```python
from build123d import *

# Parameters (mm, degrees)
SKETCH1_R           = 12.7
SKETCH1_R_2         = 1.35255
BOSS_EXTRUDE1_DEPTH = 4.445
SKETCH2_R           = 6.35
CUT_EXTRUDE1_DEPTH  = 0.762
CUT_EXTRUDE4_DEPTH  = 1.778
SKETCH6_R           = 1.8288
CUT_EXTRUDE5_DEPTH  = 2.905


with BuildPart() as part:
    # Sketch1 → Boss-Extrude1 (new body)
    with BuildSketch(Plane(origin=(0, 0, 0), x_dir=(0, 0, -1), z_dir=(1, 0, 0))):
        Circle(SKETCH1_R)
        with Locations((0, 9.779)):
            Circle(SKETCH1_R_2, mode=Mode.SUBTRACT)
        with Locations((6.914797213, 6.914797213)):
            Circle(SKETCH1_R_2, mode=Mode.SUBTRACT)
        with Locations((9.779, 0)):
            Circle(SKETCH1_R_2, mode=Mode.SUBTRACT)
        with Locations((6.914797213, -6.914797213)):
            Circle(SKETCH1_R_2, mode=Mode.SUBTRACT)
        with Locations((0, -9.779)):
            Circle(SKETCH1_R_2, mode=Mode.SUBTRACT)
        with Locations((-6.914797213, -6.914797213)):
            Circle(SKETCH1_R_2, mode=Mode.SUBTRACT)
        with Locations((-9.779, 0)):
            Circle(SKETCH1_R_2, mode=Mode.SUBTRACT)
        with Locations((-6.914797213, 6.914797213)):
            Circle(SKETCH1_R_2, mode=Mode.SUBTRACT)
    extrude(amount=BOSS_EXTRUDE1_DEPTH)

    # Sketch2 → Cut-Extrude1 (cut)
    with BuildSketch(Plane(origin=(4.445, 0, 0), x_dir=(0, 0, -1), z_dir=(1, 0, 0))):
        Circle(SKETCH2_R)
    extrude(amount=-CUT_EXTRUDE1_DEPTH, mode=Mode.SUBTRACT)

    # Sketch5 → Cut-Extrude4 (cut)
    with BuildSketch(Plane(origin=(3.683, 0, 0), x_dir=(0, 0, -1), z_dir=(1, 0, 0))):
        Polygon((-2.305627782, 3.948070989), (-4.571943663, -0.022696736), (-2.266315881, -3.970767725), (2.305627782, -3.948070989), (4.571943663, 0.022696736), (2.266315881, 3.970767725), align=None)
    extrude(amount=-CUT_EXTRUDE4_DEPTH, mode=Mode.SUBTRACT)

    # Sketch6 → Cut-Extrude5 (cut, through all)
    with BuildSketch(Plane(origin=(1.905, 0, 0), x_dir=(0, 0, -1), z_dir=(1, 0, 0))):
        Circle(SKETCH6_R)
    extrude(amount=-CUT_EXTRUDE5_DEPTH, mode=Mode.SUBTRACT)


solid = part.part
```
Model file for the job. Use its own axes, mm. A direction names the side the tool comes from. Round coordinates to 2 decimals unless told otherwise and drop trailing zeros. Loops run counter-clockwise (first coordinate to the right, second up) from the corner with the lowest first, then second, coordinate; pieces in that order, holes last. Notation, with made-up numbers: M 48,77.25 L 52,77.25 A25 cw 52,112.25 Z; hole C 48.5,-16.75 d3. An arc over 180 degrees is marked long. Put each result on its own line as item: value. Start each with the question number.
Item 1: Drill centre lines: line 1 along Z through (x, y) = (1.25, 6.75); line 2 along Z through (x, y) = (1.55, 7); line 3 along Y through (x, z) = (0.95, -0.5). Where is each one in solid material? Low to high.
Item 2: 3-axis set-ups, long thin cutter, end or side, ignore diameter. For faces 5 (the face through (2.806, 1.99, 3.423)), 6 (the face through (0, 0, -3)): which of +Z, -Z, +X, -X, +Y, -Y reach the whole face in a straight line?
Item 3: Cut at D-D (y = 4.75). List the corners of the cut face in (x, z) (3 decimals).
Item 4: Drop flat-ended pins along their axis: P1, Ø10, axis at y = -0.5, z = 0, coming from the +X side; P2, Ø1.5, axis at x = 3, y = 4.5, coming from the -Z side; P3, Ø2, axis at x = 2, y = 9.5, coming from the +Z side. Give the stop position or say it passes through.
Item 5: Mould opens along Y. For faces 1 (the face through (4.445, 6, -3)), 2 (the face through (2.19, -12.4, 2.75)), 3 (the face through (2.19, 0.41, -11.07)), 4 (the face through (2.806, -1.969, 3.435)) say: released by +Y, released by -Y, zero draft, split by the parting line, or undercut.
Item 6: Cut at B-B (z = 0). List the corners of the cut face in (x, y) (3 decimals).
Item 7: Cut at C-C (x = 3). Give the number of separate pieces and of enclosed holes in the cut face, then the cut area to 3 significant figures.
Item 8: Cut at A-A (y = -8.75). List the corners of the cut face in (x, z) (3 decimals).
Answer block:
1. line 1: -10.76 to -8.26, -5.57 to 5.57, 8.26 to 10.76
1. line 2: -10.6 to -8.26, -5.56 to 5.56, 8.26 to 10.6
1. line 3: -12.69 to -11.04, -8.52 to -1.76, 1.76 to 8.52, 11.04 to 12.69
2. face 5: +X
2. face 6: +Z, -Z, -X, +Y, -Y
3. outline: M 0,-11.778 L 4.445,-11.778 L 4.445,-4.214 L 3.683,-4.214 L 3.683,4.214 L 4.445,4.214 L 4.445,11.778 L 0,11.778 Z
4. P1: x = 3.68
4. P2: z = -12.13
4. P3: z = 9.44
5. face 1: zero draft
5. face 2: split by the parting line
5. face 3: undercut
5. face 4: undercut
6. outline: M 0,-12.7 L 4.445,-12.7 L 4.445,-11.132 L 0,-11.132 Z; M 0,-8.426 L 4.445,-8.426 L 4.445,-6.35 L 3.683,-6.35 L 3.683,-3.96 L 1.905,-3.96 L 1.905,-1.829 L 0,-1.829 Z; M 0,1.829 L 1.905,1.829 L 1.905,3.96 L 3.683,3.96 L 3.683,6.35 L 4.445,6.35 L 4.445,8.426 L 0,8.426 Z; M 0,11.132 L 4.445,11.132 L 4.445,12.7 L 0,12.7 Z
7. separate pieces: 1
7. enclosed holes: 9
7. area: 406 mm2
8. outline: M 0,-9.205 L 4.445,-9.205 L 4.445,-0.878 L 0,-0.878 Z; M 0,0.878 L 4.445,0.878 L 4.445,9.205 L 0,9.205 Z
